Print and shaded views of the part. All mm, measured from the part's lowest x, y and z. Coordinates: 2 decimals unless noted, no trailing zeros. Order: outer loops, then holes, each group sorted by start corner. A loop starts at its lowest first (then second) coordinate and runs counter-clockwise, first axis right, second up. Notation, with made-up numbers: (37, -36.75) -> (71, -36.75) arc R28 cw to (71, -17.75) -> close; hole circle Ø11 at (17.5, 34.25). An arc over 180 degrees is marked (long way). Use one line per item in the form item = value. Start each with the question number.
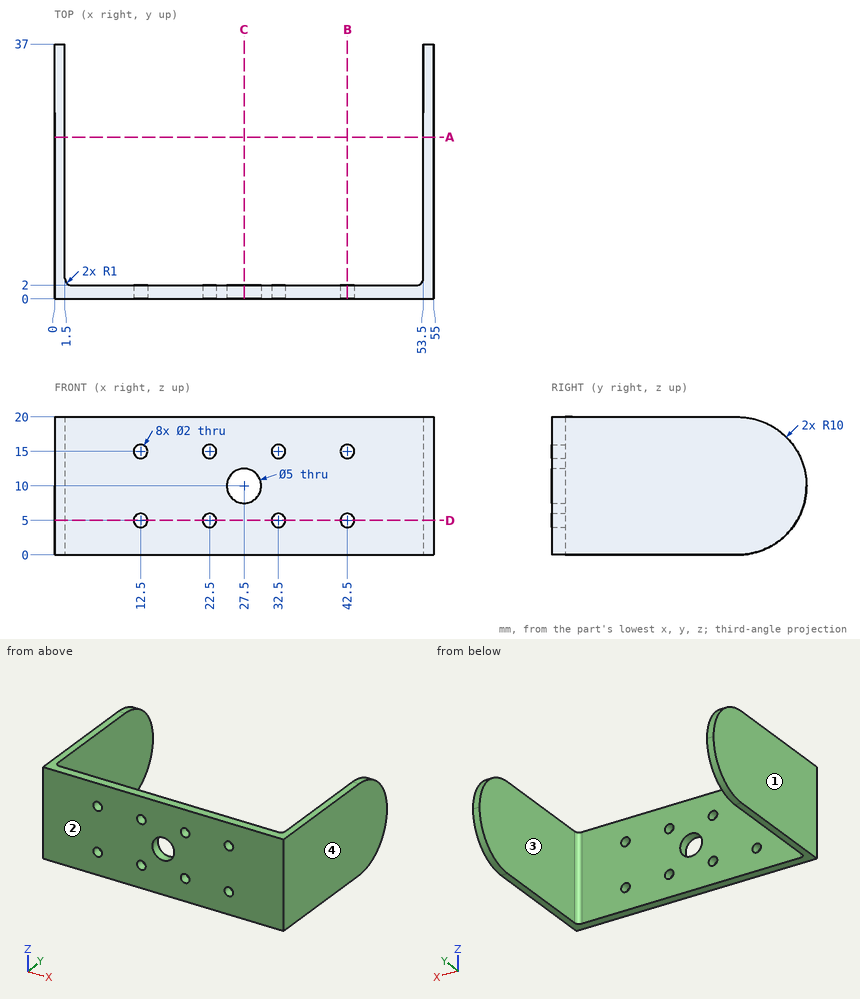
1) Two-plate mould, pull along X, no slides. Class the marked faces 1, 2, 3 and 4: released by +X, released by -X, zero draft, split by the parting line, or undercut.
2) Probe L1, parallel to X at y = 1.55, z = 5; L2, parallel to Z at x = 32.5, y = 0.7; L3, parallel to X at y = 20.5, z = 3.25. List the from-to ranges inside material, lowest first.
3) Cut at B-B on x = 42.5. Give the cut face in (y, z).
4) Cut at C-C on x = 27.5. Give the cut face in (y, z), then the cut area to 3 significant figures.
5) Drop flat-ended pins along their axis: P1, Ø1.2, axis at x = 22.5, z = 5, coming from the +Y side; P2, Ø3, axis at x = 32.5, z = 15, coming from the +Y side; P3, Ø8, axis at x = 49, z = 12, coming from the +Y side. Give the stop position or say it passes through.
6) Cut at D-D on z = 5. Give the cut face in (x, y), then the cut area to 3 significant figures.
7) Cut at A-A on y = 23.5. Give the cut face in (x, z), then the cut area to 3 significant figures.
Values follow:
q1.face_1 = released by -X
q1.face_2 = zero draft
q1.face_3 = undercut
q1.face_4 = released by +X
q2.L1 = 0 to 11.5, 13.5 to 21.5, 23.5 to 31.5, 33.5 to 41.5, 43.5 to 55
q2.L2 = 0 to 4, 6 to 14, 16 to 20
q2.L3 = 0 to 1.5, 53.5 to 55
q3.outline = (0, 0) -> (2, 0) -> (2, 4) -> (0, 4) -> close; (0, 6) -> (2, 6) -> (2, 14) -> (0, 14) -> close; (0, 16) -> (2, 16) -> (2, 20) -> (0, 20) -> close
q4.outline = (0, 0) -> (2, 0) -> (2, 7.5) -> (0, 7.5) -> close; (0, 12.5) -> (2, 12.5) -> (2, 20) -> (0, 20) -> close
q4.area = 30.0 mm^2
q5.P1 = through
q5.P2 = 2
q5.P3 = 2.13
q6.outline = (0, 0) -> (11.5, 0) -> (11.5, 2) -> (2.5, 2) arc R1 cw to (1.5, 3) -> (1.5, 35.66) -> (0, 35.66) -> close; (13.5, 0) -> (21.5, 0) -> (21.5, 2) -> (13.5, 2) -> close; (23.5, 0) -> (31.5, 0) -> (31.5, 2) -> (23.5, 2) -> close; (33.5, 0) -> (41.5, 0) -> (41.5, 2) -> (33.5, 2) -> close; (43.5, 0) -> (55, 0) -> (55, 35.66) -> (53.5, 35.66) -> (53.5, 3) arc R1 cw to (52.5, 2) -> (43.5, 2) -> close
q6.area = 195 mm^2
q7.outline = (0, 0) -> (1.5, 0) -> (1.5, 20) -> (0, 20) -> close; (53.5, 0) -> (55, 0) -> (55, 20) -> (53.5, 20) -> close
q7.area = 60.0 mm^2
